Read the model definition and answer for the solid it produces. Units are mm, in the model's axes. Face numbers are marked on the shaded views. A direction names the side the tool comes from. Round coordinates to 2 decimals unless told otherwise and drop trailing zeros. Order: outer loops, then holes, each group sorted by start corner. A loop starts at its lowest first (then second) coordinate and runs counter-clockwise, first axis right, second up.
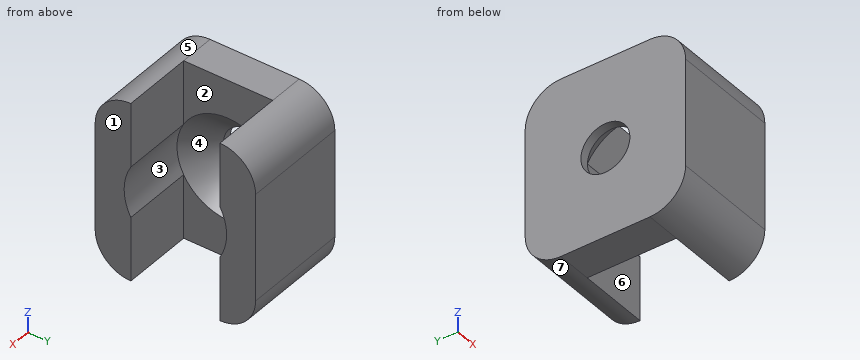
from build123d import *

# Parameters (mm, degrees)
ESQUISSE1_W             = 20
ESQUISSE1_H             = 18
BOSS_EXTRU_1_DEPTH      = 12
ESQUISSE2_W             = 8
ESQUISSE2_H             = 10
ENL_V_MAT_EXTRU_1_DEPTH = 21
ESQUISSE3_R             = 5.75
ENL_V_MAT_EXTRU_2_DEPTH = 8
CONG_2_R                = 4


with BuildPart() as part:
    # Esquisse1 → Boss.-Extru.1 (new body)
    with BuildSketch(Plane(origin=(8.078830023, 0, 0), x_dir=(0, 0, -1), z_dir=(1, 0, 0))):
        with Locations((-10, 10.8)):
            Rectangle(ESQUISSE1_W, ESQUISSE1_H)
    extrude(amount=-BOSS_EXTRU_1_DEPTH)

    # Esquisse2 → Enlèv. mat.-Extru.1 (cut, through all)
    with BuildSketch(Plane(origin=(0, 0, 0), x_dir=(-1, 0, 0), z_dir=(0, 0, -1))):
        with Locations((-4.078830023, 10.8)):
            Rectangle(ESQUISSE2_W, ESQUISSE2_H)
    extrude(amount=-ENL_V_MAT_EXTRU_1_DEPTH, mode=Mode.SUBTRACT)

    # Esquisse3 → Enlèv. mat.-Extru.2 (cut)
    with BuildSketch(Plane(origin=(8.078830023, 0, 0), x_dir=(0, 0, -1), z_dir=(1, 0, 0))):
        with Locations((-9.999999999, 10.8)):
            Circle(ESQUISSE3_R)
    extrude(amount=-ENL_V_MAT_EXTRU_2_DEPTH, mode=Mode.SUBTRACT)

    # Esquisse5 → Enlèvement de matière-Révolution1 (revolve, cut)
    with BuildSketch(Plane(origin=(0, 0, 10), x_dir=(-1, 0, 0), z_dir=(0, 0, -1)), mode=Mode.PRIVATE) as enl_vement_de_mati_re_r_volution1_sk:
        Polygon((-0.078830023, 16.55), (-0.078830023, 10.8), (3.921169977, 10.8), (3.921169977, 13.55), (2.921169977, 13.55), align=None)
    revolve(enl_vement_de_mati_re_r_volution1_sk.sketch.rotate(Axis((0.078830023, 10.8, 10), (-1, 0, 0)), 29.591845803), axis=Axis((0.078830023, 10.8, 10), (-1, 0, 0)), mode=Mode.SUBTRACT)  # turned: the seam where the file's is

    # Congé2
    cong_2_edges = [part.edges().sort_by_distance(p)[0] for p in [
        (2.078830023, 1.8, 20),
        (2.078830023, 19.8, 0),
        (2.078830023, 1.8, 0),
        (2.078830023, 19.8, 20),
    ]]
    fillet(cong_2_edges, radius=CONG_2_R)


solid = part.part
Q1. For the marked faces 1, 2 and 3, determine the directions among +Z, -Z, +X, -X, +Y, -Y from which every point of the face is accessible in a straight line to the end or side of a thin tool.
Outcome:
face 1: +Z, -Z, +X, +Y, -Y
face 2: +Z, -Z, +X
face 3: +X
Q2. A cutting plane is placed at B-B, the plane z = 10. Give the vertices of the cut face in (x, y), plus the area to 3 significant figures.
Outcome:
outline: (-3.92, 1.8) - (8.08, 1.8) - (8.08, 5.05) - (0.08, 5.05) - (-2.92, 8.05) - (-3.92, 8.05) - close; (-3.92, 13.55) - (-2.92, 13.55) - (0.08, 16.55) - (8.08, 16.55) - (8.08, 19.8) - (-3.92, 19.8) - close
area: 93.0 mm2
Q3. A cutting plane is placed at C-C, the plane x = 2.5. Give the vertices of the cut face in (y, z).
Outcome:
outline: (1.8, 4) arc R4 ccw to (5.8, 0) - (5.8, 7.16) arc R5.75 cw to (5.8, 12.84) - (5.8, 20) arc R4 ccw to (1.8, 16) - close; (15.8, 0) arc R4 ccw to (19.8, 4) - (19.8, 16) arc R4 ccw to (15.8, 20) - (15.8, 12.84) arc R5.75 cw to (15.8, 7.16) - close
Q4. A cutting plane is placed at A-A, the plane y = 10.8. Give the vertices of the cut face in (x, z), plus the area to 3 significant figures.
Outcome:
outline: (-3.92, 0) - (0.08, 0) - (0.08, 4.25) - (-2.92, 7.25) - (-3.92, 7.25) - close; (-3.92, 12.75) - (-2.92, 12.75) - (0.08, 15.75) - (0.08, 20) - (-3.92, 20) - close
area: 49.0 mm2
Q5. For a pull along Z with two mould halves and no side action, classify the marked faces 4, 5, 6 and 7 as released by +Z, released by -Z, zero draft, split by the parting line, or undercut.
Outcome:
face 4: undercut
face 5: released by +Z
face 6: zero draft
face 7: released by -Z
Q6. Straight lines are drawn through the part: probe 1 along Z at (x, y) = (-3.7, 10.8); probe 2 along Y at (x, z) = (-3.5, 10); probe 3 along Y at (x, z) = (5.5, 5). For each, find the intervals that lie inside material, in ascending order.
Outcome:
probe 1: z = 0 to 7.25, 12.75 to 20
probe 2: y = 1.8 to 8.05, 13.55 to 19.8
probe 3: y = 1.8 to 5.8, 15.8 to 19.8
Q7. A flat-ended cylindrical pin translates along its axis: pin 1 (3.5 mm diameter, centred on y = 11, z = 2, fed in from +X). Find the tip coordinate at first contact, or state that the pin passes through.
Outcome:
pin 1: stops at x = 0.08
Q8. A cutting plane is placed at D-D, the plane x = -0.5. Give the vertices of the cut face in (y, z), plus the area to 3 significant figures.
Outcome:
outline: (1.8, 4) arc R4 ccw to (5.8, 0) - (15.8, 0) arc R4 ccw to (19.8, 4) - (19.8, 16) arc R4 ccw to (15.8, 20) - (5.8, 20) arc R4 ccw to (1.8, 16) - close; hole circle Ø10.34 at (10.8, 10)
area: 262 mm2
